Can you work these out from the model? Positions are in its coordinate system, mm. Give positions to 0.01 mm unless a question says otherwise; leave off trailing zeros. Order: outer loops, then holes, each group sorted by start corner. A loop starts at its lowest first (then second) coordinate and runs counter-clockwise, first axis right, second up.
Item 1: If I drill on line 1 along X through (y, z) = (0.55, -5.75); line 2 along X through (y, z) = (0.75, -5); line 3 along Y through (x, z) = (5.5, 7), over which ranges is the centre line in solid material (lowest first)?
Item 2: I want a section at D-D, the plane x = 4. Write out the boundary of the cut face in (y, z), then the cut area to 3 significant figures.
Item 3: I'm going to push flat-ended pins straight in: pin 1 Ø3 at (x, z) = (-5.1, -4.68) entering from +Y; pin 2 Ø5 at (x, z) = (1, -5) entering from +Y. Where does each tip first touch, or does it pass through?
Item 4: I want a section at A-A, the plane z = -6. Write out the boundary of the cut face in (x, y).
Item 5: I want a section at C-C, the plane z = 2.5. Write out the boundary of the cut face in (x, y).
Item 6: I want a section at B-B, the plane x = -3.5. Write out the boundary of the cut face in (y, z).
```python
from build123d import *

# Parameters (mm, degrees)
SKETCH1_W           = 19.05
SKETCH1_H           = 16.51
BOSS_EXTRUDE1_DEPTH = 1.27
SKETCH2_R           = 1.905
CUT_EXTRUDE1_DEPTH  = 1.27
SKETCH3_W           = 1.25000004
SKETCH3_H           = 1.75
BOSS_EXTRUDE2_DEPTH = 0.127


with BuildPart() as part:
    # Sketch1 → Boss-Extrude1 (new body)
    with BuildSketch(Plane(origin=(0, 0, 0), x_dir=(1, 0, 0), z_dir=(0, 1, 0))):
        with Locations((1.883228571, -1.037771429)):
            Rectangle(SKETCH1_W, SKETCH1_H)
    extrude(amount=BOSS_EXTRUDE1_DEPTH)

    # Sketch2 → Cut-Extrude1 (cut)
    with BuildSketch(Plane(origin=(0, 1.27, 0), x_dir=(1, 0, 0), z_dir=(0, 1, 0))):
        with Locations((-5.101771429, 4.677228571)):
            Circle(SKETCH2_R)
        with Locations((8.868228571, 4.677228571)):
            Circle(SKETCH2_R)
    extrude(amount=-CUT_EXTRUDE1_DEPTH, mode=Mode.SUBTRACT)

    # Sketch3 → Boss-Extrude2 (add)
    with BuildSketch(Plane(origin=(0, 1.27, 0), x_dir=(1, 0, 0), z_dir=(0, 1, 0))):
        with Locations((1.883228571, -2.448771429)):
            Rectangle(SKETCH3_W, SKETCH3_H)
    extrude(amount=BOSS_EXTRUDE2_DEPTH)


solid = part.part
```
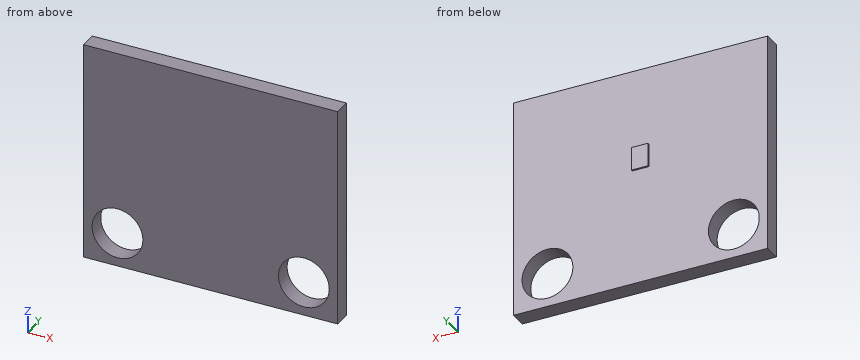
Results list:
1. line 1: x = -7.64 to -6.68, -3.53 to 7.29, 10.44 to 11.41
1. line 2: x = -7.64 to -6.98, -3.22 to 6.99, 10.75 to 11.41
1. line 3: y = 0 to 1.27
2. outline: (0, -7.22) - (1.27, -7.22) - (1.27, 9.29) - (0, 9.29) - close
2. area: 21.0 mm2
3. pin 1: passes through
3. pin 2: stops at y = 1.27
4. outline: (-7.64, 0) - (-6.47, 0) - (-6.47, 1.27) - (-7.64, 1.27) - close; (-3.73, 0) - (7.5, 0) - (7.5, 1.27) - (-3.73, 1.27) - close; (10.24, 0) - (11.41, 0) - (11.41, 1.27) - (10.24, 1.27) - close
5. outline: (-7.64, 0) - (11.41, 0) - (11.41, 1.27) - (2.51, 1.27) - (2.51, 1.4) - (1.26, 1.4) - (1.26, 1.27) - (-7.64, 1.27) - close
6. outline: (0, -7.22) - (1.27, -7.22) - (1.27, -5.71) - (0, -5.71) - close; (0, -3.65) - (1.27, -3.65) - (1.27, 9.29) - (0, 9.29) - close
